Drawing for the job (mm, zero at the part's lowest x, y, z). Coordinates: 2 decimals unless noted, no trailing zeros. Write each loop counter-clockwise with the first axis right and the second up, starting at its lowest first coordinate (ties: lowest second). Pieces come first, ordered by that corner, then holes. Notation, with made-up numbers: M 24,39 L 76,39 A11 cw 76,57 Z; hole C 78.25,46.5 d4. An arc over 180 degrees is marked long. Use a Markdown table: item, result. Add a question column.
Q1. Wall check: L1, parallel to Z at x = 28, y = 2.6; L2, parallel to Y at x = 7.5, z = 27.5. Give the ranges that are in metal, low to high. Write a range as from..to.
Q2. Pin check, flat tips, straight feed: pin 1 Ø4 at (x, z) = (12.5, 11.5) entering from +Y; pin 2 Ø17 at (x, z) = (12, 24) entering from +Y. Stop position of each tip, or through.
Q3. Slice it at B-B on z = 1. Write the cut outline in (x, y), then the cut area to 3 significant figures.
Q4. Slice it at D-D on z = 12. Write the cut outline in (x, y).
Q5. Slice it at A-A on y = 2.55. Write the cut outline in (x, z).
Q6. Mould opens along X. For the marked faces 1, 2 and 3 say: released by +X, released by -X, zero draft, split by the parting line, or undercut.
Q7. Slice it at C-C on x = 19.5. Write the cut outline in (y, z).
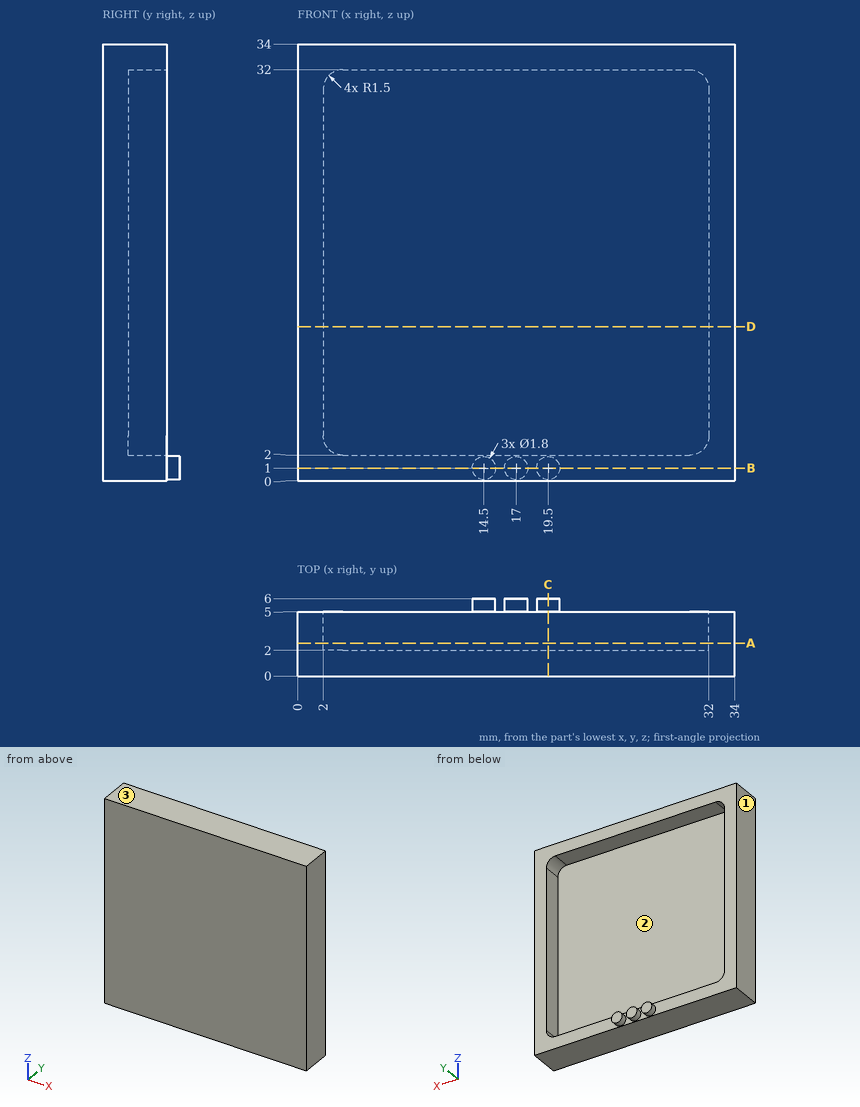
Recorded:
| question | item | result |
|---|---|---|
| 1 | L1 | 0..2, 32..34 |
| 1 | L2 | 0..2 |
| 2 | pin 1 | y = 2 |
| 2 | pin 2 | y = 5 |
| 3 | outline | M 0,0 L 34,0 L 34,5 L 20.4,5 L 20.4,6 L 18.6,6 L 18.6,5 L 17.9,5 L 17.9,6 L 16.1,6 L 16.1,5 L 15.4,5 L 15.4,6 L 13.6,6 L 13.6,5 L 0,5 Z |
| 3 | area | 175 mm² |
| 4 | outline | M 0,0 L 34,0 L 34,5 L 32,5 L 32,2 L 2,2 L 2,5 L 0,5 Z |
| 5 | outline | M 0,0 L 34,0 L 34,34 L 0,34 Z; hole M 2,3.5 A1.5 ccw 3.5,2 L 30.5,2 A1.5 ccw 32,3.5 L 32,30.5 A1.5 ccw 30.5,32 L 3.5,32 A1.5 ccw 2,30.5 Z |
| 6 | face 1 | released by -X |
| 6 | face 2 | undercut |
| 6 | face 3 | zero draft |
| 7 | outline | M 0,0 L 5,0 L 5,0.1 L 6,0.1 L 6,1.9 L 5,1.9 L 5,2 L 2,2 L 2,32 L 5,32 L 5,34 L 0,34 Z |
